For this review, take the finished solid that the model builds, in its own axes (mm). A direction names the side the tool comes from. Round coordinates to 2 decimals unless told otherwise and drop trailing zeros. Loops run counter-clockwise (first coordinate to the right, second up) from the corner with the lowest first, then second, coordinate; pieces in that order, holes last. Notation, with made-up numbers: (-5, 40) -> (4, 40) arc R14 ccw to (4, 57) -> close; hole circle Ø7 at (11.5, 33). An arc over 180 degrees is marked (long way). One line per question, with ' | ' between items. Start each with the question number.
1. Consider section B-B (z = 0). Write out the cut boundary in (x, y), and give its area (3 significant figures).
2. Consider section A-A (x = 0). Write out the cut boundary in (y, z), and give its area (3 significant figures).
3. Draft analysis for pull direction Y (two halves, no side actions). For faces 4 (the face through (51, 0, -28)), 5 (the face through (51.46, 11.02, -26.76)), 6 (the face through (51.46, 26.4, -26.76)), 7 (the face through (-62.464, 2.958, 8.201)), state which applies: pulls with the +Y half, pulls with the -Y half, needs draft (parallel to the pull), parting line crosses it, or undercut.
4. Consider section D-D (y = 39.5). Write out the cut boundary in (x, z).
5. For faces 1 (the face through (46.4, 6, 41.7)), 2 (the face through (51.46, 3.3, -26.76)), 3 (the face through (-14.718, 39.535, -46.737)), list the 3-axis set-ups (+Z, -Z, +X, -X, +Y, -Y) from which the entire face can be reached by the end or side of a thin tool; tool diameter is ignored.
6. For pin 1 Ø8 at (x, z) = (17, -40.5) entering from +Y; pin 2 Ø12 at (x, z) = (46, 22) entering from -Y; pin 3 Ø1 at (y, z) = (38, -39) entering from +X; pin 4 Ø1.5 at (y, z) = (25.5, 28.5) entering from +X, all flat-tipped, find the tip position at first contact; note any pin that passes through.
7. Wall thickness on line 1 along X through (y, z) = (10.85, 0); line 2 along X through (y, z) = (3.25, 0); line 3 along Y through (x, z) = (53, 4.5): over which ranges is each line inside the solid? List them lowest first.
8. Consider section C-C (y = 27). Write out the cut boundary in (x, z).
```python
from build123d import *


with BuildPart() as part:
    # Sketch1 → Revolve1 (revolve)
    with BuildSketch(Plane.XY, mode=Mode.PRIVATE) as revolve1_sk:
        with BuildLine():
            Line((49, 42), (63, 42))
            Line((63, 42), (63, 22))
            Line((63, 22), (62.2, 22))
            Line((62.2, 22), (62.2, 6))
            Line((62.2, 6), (63, 6))
            Line((63, 6), (63, 0))
            Line((63, 0), (58, 0))
            Line((58, 0), (58, 6.5))
            ThreePointArc((58, 6.5), (56.5, 8), (58, 9.5))
            Line((58, 9.5), (58, 12.5))
            ThreePointArc((58, 12.5), (56.5, 14), (58, 15.5))
            Line((58, 15.5), (58, 37))
            Line((58, 37), (49, 37))
            Line((49, 37), (49, 42))
        make_face()
    revolve(revolve1_sk.sketch.rotate(Axis((0, 0, 0), (0, 1, 0)), 90), axis=Axis((0, 0, 0), (0, 1, 0)))


solid = part.part
```
Answer block:
1) outline: (-63, 0) -> (-58, 0) -> (-58, 6.5) arc R1.5 ccw to (-58, 9.5) -> (-58, 12.5) arc R1.5 ccw to (-58, 15.5) -> (-58, 37) -> (-49, 37) -> (-49, 42) -> (-63, 42) -> (-63, 22) -> (-62.2, 22) -> (-62.2, 6) -> (-63, 6) -> close; (49, 37) -> (58, 37) -> (58, 15.5) arc R1.5 ccw to (58, 12.5) -> (58, 9.5) arc R1.5 ccw to (58, 6.5) -> (58, 0) -> (63, 0) -> (63, 6) -> (62.2, 6) -> (62.2, 22) -> (63, 22) -> (63, 42) -> (49, 42) -> close | area: 499 mm2
2) outline: (0, -63) -> (6, -63) -> (6, -62.2) -> (22, -62.2) -> (22, -63) -> (42, -63) -> (42, -49) -> (37, -49) -> (37, -58) -> (15.5, -58) arc R1.5 ccw to (12.5, -58) -> (9.5, -58) arc R1.5 ccw to (6.5, -58) -> (0, -58) -> close; (0, 58) -> (6.5, 58) arc R1.5 ccw to (9.5, 58) -> (12.5, 58) arc R1.5 ccw to (15.5, 58) -> (37, 58) -> (37, 49) -> (42, 49) -> (42, 63) -> (22, 63) -> (22, 62.2) -> (6, 62.2) -> (6, 63) -> (0, 63) -> close | area: 499 mm2
3) face 4: pulls with the -Y half | face 5: undercut | face 6: undercut | face 7: needs draft
4) outline: circle Ø126 at (0, 0); hole circle Ø98 at (0, 0)
5) face 1: none | face 2: -Y | face 3: +Y, -Y
6) pin 1: passes through | pin 2: stops at y = 6.89 | pin 3: stops at x = 49.87 | pin 4: stops at x = 56.56
7) line 1: x = -62.2 to -58, 58 to 62.2 | line 2: x = -63 to -58, 58 to 63 | line 3: y = 37 to 42
8) outline: circle Ø126 at (0, 0); hole circle Ø116 at (0, 0)
